Geometry: final body of the model. Coordinates: model frame, mm. A direction names the side the tool comes from. Give positions to 0.01 mm unless a question says otherwise; leave off trailing zeros. Order: outer loops, then holes, each group sorted by start corner. A loop starts at its lowest first (then second) coordinate and runs counter-clockwise, first axis right, second up. Notation, with made-up numbers: (22, 48) -> (33, 48) arc R5 ccw to (33, 57) -> close; hole circle Ø6 at (61.25, 78.25). An arc over 180 degrees is marked (long way). Write item = value, one per line.
```python
from build123d import *

# Parameters (mm, degrees)
EXTRUDE_1_DEPTH = 4.7
SKETCH_2_W      = 0.5
SKETCH_2_H      = 0.3
EXTRUDE_2_DEPTH = 2
SKETCH_3_W      = 0.5
SKETCH_3_H      = 0.3
EXTRUDE_3_DEPTH = 11


with BuildPart() as part:
    # 草图1 → 凸台-拉伸1 (new body)
    with BuildSketch(Plane(origin=(0, 0, 0), x_dir=(1, 0, 0), z_dir=(0, 1, 0))):
        with BuildLine():
            Line((-2.35, 0), (2.35, 0))
            Line((2.35, 0), (2.35, 1.15))
            ThreePointArc((2.35, 1.15), (0, 3.5), (-2.35, 1.15))
            Line((-2.35, 1.15), (-2.35, 0))
        make_face()
    extrude(amount=EXTRUDE_1_DEPTH)

    # 草图2 → 凸台-拉伸2 (add)
    with BuildSketch(Plane.XZ):
        with Locations((1.25, -1.15)):
            Rectangle(SKETCH_2_W, SKETCH_2_H)
        with Locations((0, -1.15)):
            Rectangle(SKETCH_2_W, SKETCH_2_H)
        with Locations((-1.25, -1.15)):
            Rectangle(SKETCH_2_W, SKETCH_2_H)
    extrude(amount=EXTRUDE_2_DEPTH)

    # 草图3 → 凸台-拉伸3 (add)
    with BuildSketch(Plane.XY.offset(-1)):
        with Locations((0, -2.15)):
            Rectangle(SKETCH_3_W, SKETCH_3_H)
        with Locations((-1.25, -2.15)):
            Rectangle(SKETCH_3_W, SKETCH_3_H)
        with Locations((1.25, -2.15)):
            Rectangle(SKETCH_3_W, SKETCH_3_H)
    extrude(amount=-EXTRUDE_3_DEPTH)


solid = part.part
```
1) Section query B-B (z = -8.25). Output: boundary loops of the cut face in (x, y), plus the area to 3 significant figures.
Check sheet entries:
outline = (-1.5, -2.3) -> (-1, -2.3) -> (-1, -2) -> (-1.5, -2) -> close; (-0.25, -2.3) -> (0.25, -2.3) -> (0.25, -2) -> (-0.25, -2) -> close; (1, -2.3) -> (1.5, -2.3) -> (1.5, -2) -> (1, -2) -> close
area = 0.450 mm²
2) Line query: line 1 (Y direction, x = 1.3, z = -2); line 2 (Z direction, x = 0.15, y = -1.25); line 3 (Y direction, x = 1.15, z = -5.5). Output: solid intervals per line, ascending. Write a range as from..to.
Check sheet entries:
line_1 = -2.3..-2, 0..4.7
line_2 = -1.3..-1
line_3 = -2.3..-2
3) Section query D-D (z = -3). Output: boundary loops of the cut face in (x, y).
Check sheet entries:
outline = (-1.5, -2.3) -> (-1, -2.3) -> (-1, -2) -> (-1.5, -2) -> close; (-1.45, 0) -> (1.45, 0) -> (1.45, 4.7) -> (-1.45, 4.7) -> close; (-0.25, -2.3) -> (0.25, -2.3) -> (0.25, -2) -> (-0.25, -2) -> close; (1, -2.3) -> (1.5, -2.3) -> (1.5, -2) -> (1, -2) -> close
4) Mould query, pull axis Y, two halves, no side actions, for faces 1 (the face through (0, 0, -2)), 2 (the face through (0, 4.7, -1)), 3 (the face through (-2.35, 2.3, -0.6)). Classes: +Y half, -Y half, draft (parallel to the pull), parting line (faces both ways), or undercut.
Check sheet entries:
face_1 = undercut
face_2 = +Y half
face_3 = draft
5) Section query C-C (x = 0). Output: boundary loops of the cut face in (y, z).
Check sheet entries:
outline = (-2.3, -12) -> (-2, -12) -> (-2, -1.3) -> (0, -1.3) -> (0, -3.5) -> (4.7, -3.5) -> (4.7, 0) -> (0, 0) -> (0, -1) -> (-2.3, -1) -> close
6) Section query A-A (y = -0.5). Output: boundary loops of the cut face in (x, z), plus the area to 3 significant figures.
Check sheet entries:
outline = (-1.5, -1.3) -> (-1, -1.3) -> (-1, -1) -> (-1.5, -1) -> close; (-0.25, -1.3) -> (0.25, -1.3) -> (0.25, -1) -> (-0.25, -1) -> close; (1, -1.3) -> (1.5, -1.3) -> (1.5, -1) -> (1, -1) -> close
area = 0.450 mm²
7) Reachability of faces 4 (the face through (0.05, 2.32, -3.5)), 5 (the face through (2.35, 2.3, -0.6)) from +Z, -Z, +X, -X, +Y, -Y: full face, straight path, thin tool, end or side. Return the list, or none.
Check sheet entries:
face_4 = -Z, +Y
face_5 = +Z, -Z, +X, +Y, -Y
8) First-contact query: P1, Ø0.6, axis at x = 0, y = -1.5, coming from the -Z side; P2, Ø0.6, axis at x = 1, z = -6.5, coming from the +Y side; P3, Ø1.5, axis at x = 1.5, y = -1.5, coming from the -Z side; P4, Ø1.2, axis at y = -1.5, z = -4.5, coming from the -X side. Flat tips, straight axial feed; report the tip coordinate or a pass-through.
Check sheet entries:
P1 = -1.3
P2 = -2
P3 = -12
P4 = -1.5
